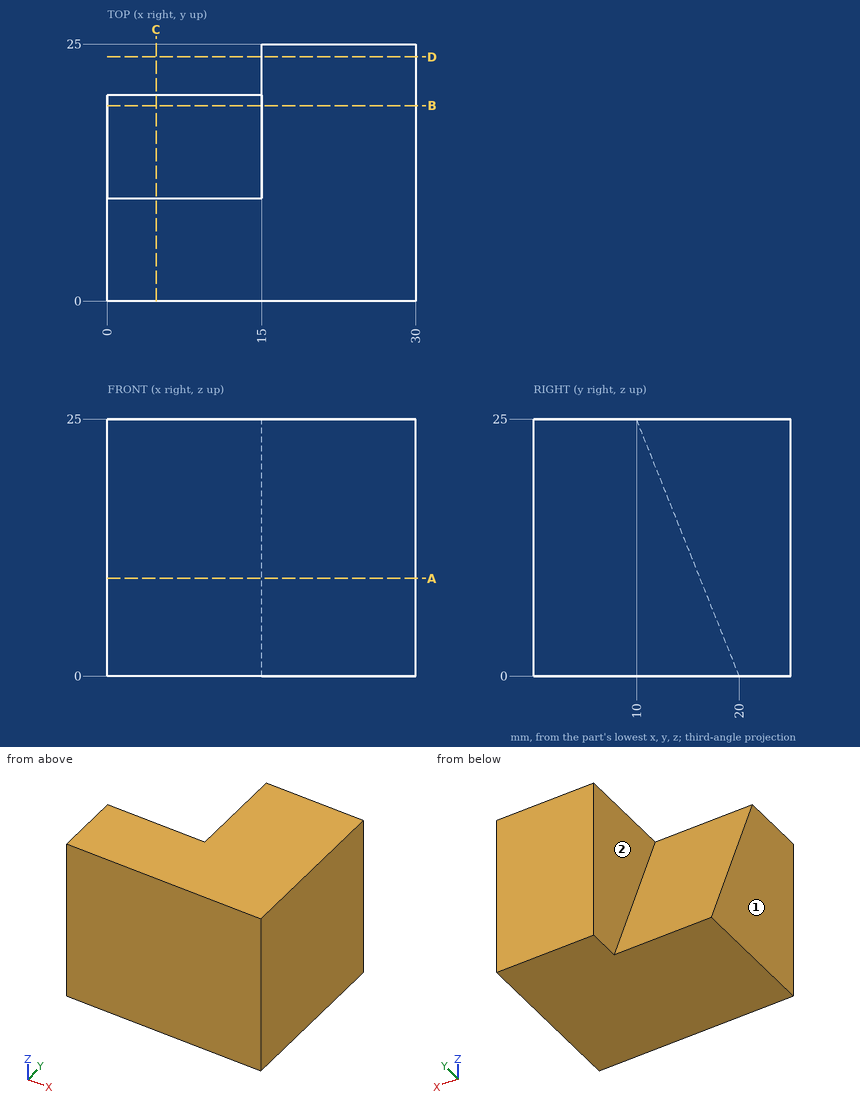
Verification items for this drawing (mm, ordinates from the low corner). A direction names the side the tool comes from. Coordinates: 2 decimals unless noted, no trailing zeros. Loops run counter-clockwise (first coordinate to the right, second up) from the corner with the lowest first, then second, coordinate; pieces in that order, holes last. Notation, with made-up numbers: (5, 48.25) -> (37, 48.25) arc R21 cw to (37, 84.25) -> close; hole circle Ø8 at (64.5, -31). An arc over 180 degrees is marked (long way). Put each result on its own line as item: value.
1. Section check D-D, the plane y = 23.75. Record the boundary of the cut face in (x, z), then the cut area to 3 significant figures.
Result set:
outline: (15, 0) -> (30, 0) -> (30, 25) -> (15, 25) -> close
area: 375 mm^2
2. Section check B-B, the plane y = 19. Record the boundary of the cut face in (x, z).
Result set:
outline: (0, 0) -> (30, 0) -> (30, 25) -> (15, 25) -> (15, 2.5) -> (0, 2.5) -> close
3. Thickness scan on line 1 (X direction, y = 22.5, z = 17.75); line 2 (Y direction, x = 12, z = 6); line 3 (Y direction, x = 4.25, z = 22.75). Record the ranges inside material, lowest first.
Result set:
line 1: x = 15 to 30
line 2: y = 0 to 17.6
line 3: y = 0 to 10.9
4. Gauge pin test, flat ends, axial feed: P1, Ø6, axis at x = 8.5, y = 17, coming from the +Z side; P2, Ø10, axis at x = 4.5, z = 12, coming from the -Y side. Record the tip position at first contact, or that the pin passes through.
Result set:
P1: stops at z = 15
P2: stops at y = 0
5. Section check C-C, the plane x = 4.75. Record the boundary of the cut face in (y, z).
Result set:
outline: (0, 0) -> (20, 0) -> (10, 25) -> (0, 25) -> close
6. Tool access check on the marked faces 1 and 2. Record the directions out of +Z, -Z, +X, -X, +Y, -Y that give a thin tool (end or side, any length) a straight path to the whole face; none if there is none.
Result set:
face 1: +Z, -Z, -X, +Y, -Y
face 2: +Z, -X, +Y
7. Section check A-A, the plane z = 9.5. Record the boundary of the cut face in (x, y), then the cut area to 3 significant figures.
Result set:
outline: (0, 0) -> (30, 0) -> (30, 25) -> (15, 25) -> (15, 16.2) -> (0, 16.2) -> close
area: 618 mm^2
